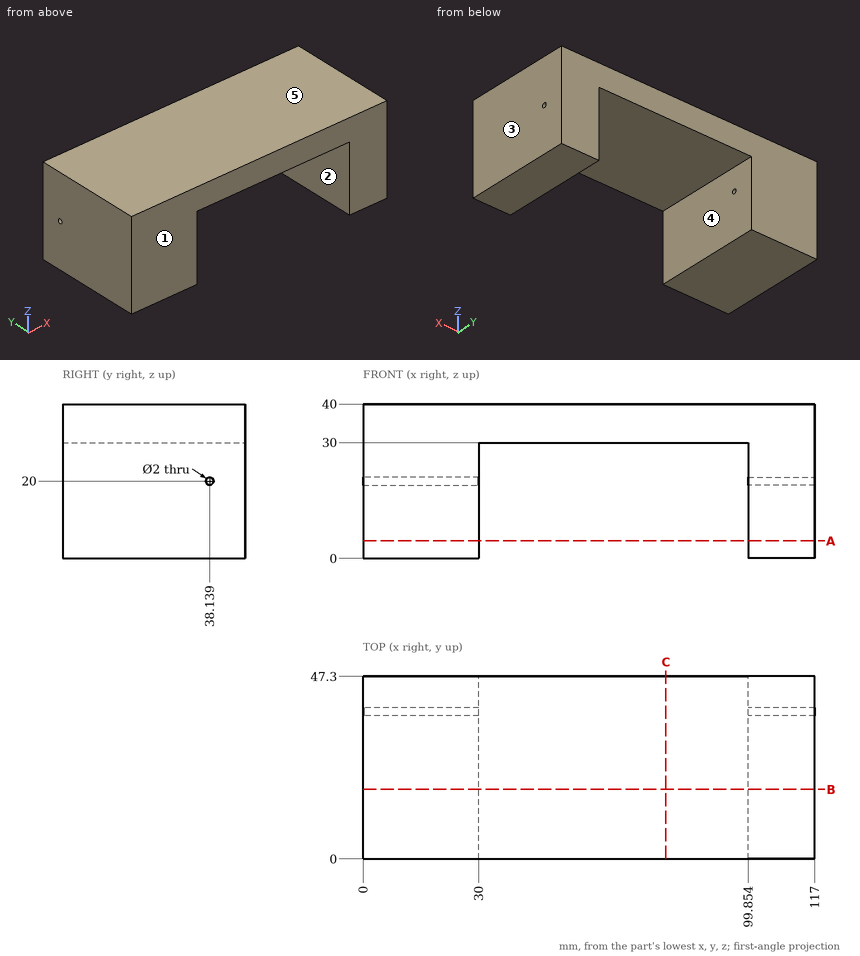
Answer from the drawing. Dimensions are ordinates in mm from the lowest x, y and z of the part. A direction names the side the tool comes from. Coordinates: 2 decimals unless noted, no trailing zeros. Order: outer loops, then holes, each group sorted by start corner. A loop starts at its lowest first (then second) coordinate and runs counter-clockwise, first axis right, second up. Notation, with made-up numbers: (-13, 50.5) - (37, 50.5) arc R31 ccw to (37, 86.5) - close; hole circle Ø7 at (9, 58). An arc over 180 degrees is marked (long way). Answer as a JSON object with one key per item and string values. Group by question number.
Item 1: Section C-C (x = 78.5) is taken. Give the vertices of the cut face in (y, z), plus the area to 3 significant figures.
Item 2: Consider probe 1 along X at (y, z) = (29, 26.5); probe 2 along Y at (x, z) = (8, 20); probe 3 along Z at (x, y) = (97, 13.5). Determine where each line is inside the solid, lowest interval first. Write a range as from..to.
Item 3: Section A-A (z = 4.5) is taken. Give the vertices of the cut face in (x, y).
Item 4: A flat-ended cylindrical pin translates along its axis: P1, Ø1.8, axis at y = 38.14, z = 20, coming from the -X side. Find the tip coordinate at first contact, or state that the pin passes through.
Item 5: Section B-B (y = 18) is taken. Give the vertices of the cut face in (x, z), plus the area to 3 significant figures.
Item 6: The mould has two halves that part along X. Classify the marked faces 3, 4 and 5: +X half, -X half, draft (parallel to the pull), parting line (faces both ways), or undercut.
Item 7: A tool of negligible diameter and unlimited length cuts with its end or side. For the marked faces 1 and 2, from which of +Z, -Z, +X, -X, +Y, -Y can it reach the whole face along a straight path? Write none if from no direction.
Results are:
{
 "1": {"outline": "(0, 30) - (47.3, 30) - (47.3, 40) - (0, 40) - close", "area": "473 mm^2"},
 "2": {"probe 1": "x = 0..30, 99.85..117", "probe 2": "y = 0..37.14, 39.14..47.3", "probe 3": "z = 30..40"},
 "3": {"outline": "(0, 0) - (30, 0) - (30, 47.3) - (0, 47.3) - close; (99.85, 0) - (117, 0) - (117, 47.3) - (99.85, 47.3) - close"},
 "4": {"P1": "passes through"},
 "5": {"outline": "(0, 0) - (30, 0) - (30, 30) - (99.85, 30) - (99.85, 0) - (117, 0) - (117, 40) - (0, 40) - close", "area": "2,580 mm^2"},
 "6": {"face 3": "+X half", "face 4": "undercut", "face 5": "draft"},
 "7": {"face 1": "+Z, -Z, +X, -X, -Y", "face 2": "-Z, +Y, -Y"}
}
